Autodesk Inventor part; units mm, degrees
ref_plane "YZ Plane" through (0, 0, 0) normal (1, 0, 0) x (0, 1, 0)
ref_plane "XZ Plane" through (0, 0, 0) normal (0, 1, 0) x (-1, 0, 0)
ref_plane "XY Plane" through (0, 0, 0) normal (0, 0, 1) x (1, 0, 0)
sketch "Schizzo1" plane through (0, 0, 0) normal (0, 0, 1) x (1, 0, 0)
  line L0 (50, -12.5) -> (-50, -12.5)
  line L1 (-50, -12.5) -> (-50, 12.5)
  line L2 (-50, 12.5) -> (50, 12.5)
  line L3 (50, 12.5) -> (50, -12.5)
  line L4 (50, -12.5) -> (-50, 12.5) construction
  line L5 (-50, -12.5) -> (50, 12.5) construction
  point P0 (0, 0)
  dimension "d0" = 100
  dimension "d1" = 25
extrude "Estrusione1" add sketch "Schizzo1" along normal blind 15
sketch "Schizzo2" plane through (-50, 12.5, 0) normal (0, 1, 0) x (1, 0, 0)
  line L0 (50, 0) -> (50, 1)
  line L1 (50, 0) -> (51, 0) construction
  circle A0 centre (50, 1) radius 9.5
  dimension "d4" = 1
  dimension "d5" = 90
  dimension "d6" = 19
extrude "Estrusione2" cut sketch "Schizzo2" against normal blind 5
sketch "Schizzo3" plane through (-50, 7.5, 0) normal (0, 1, 0) x (1, 0, 0)
  line L0 (50, 0) -> (50, 1)
  line L1 (50, 0) -> (51, 0) construction
  circle A0 centre (50, 1) radius 4
  dimension "d9" = 1
  dimension "d10" = 90
  dimension "d11" = 8
extrude "Estrusione3" cut sketch "Schizzo3" against normal blind 20
sketch "Schizzo4" plane through (0, 0, 15) normal (0, 0, 1) x (1, 0, 0)
  line L0 (-25, 0) -> (25, 0)
  line L1 (-25, 0) -> (25, 0) construction
  line L2 (50, 12.5) -> (-50, 12.5)
  point P0 (0, 0)
  point P1 (0, 0)
  dimension "d14" = 50
  dimension "d15" = 0
hole "Foro1" at (-25, 0, 15) at (25, 0, 15) direction (0, 0, -1) diameter 5.9 end through all
sketch "Schizzo5" plane through (-50, 12.5, 15) normal (0, 1, 0) x (1, 0, 0)
  circle A0 centre (50, 15) radius 23
  line L0 (100, 0) -> (0, 0)
  line L1 (67.4356, 0) -> (32.5644, 0)
  point P0 (50, 15)
  dimension "d23" = 46
extrude "Estrusione4" add sketch "Schizzo5" against normal blind 25 contours L0 A0 picked at (45.5796, -1.264)
properties part number "20_Base_Sopra" material "PLA(Stampato)(D0,646)"
Part model, mm, in its own coordinate system. A direction names the side the tool comes from. Give positions to 0.01 mm unless a question says otherwise; leave off trailing zeros. Order: outer loops, then holes, each group sorted by start corner. A loop starts at its lowest first (then second) coordinate and runs counter-clockwise, first axis right, second up. Notation, with made-up numbers: M 40,-10.5 L 49,-10.5 A12 cw 49,6.5 Z; hole C 82,44.5 d9. An arc over 180 degrees is marked long. Use a Markdown table: item, result. Add a question column.
(1) Saw through at D-D, the plane y = 8.5. Give the cut face in (x, z).
(2) Saw through at B-B, the plane x = 25. Give the cut face in (y, z).
(3) Saw through at C-C, the plane z = 11. Give the cut face in (x, y), and give its area (3 significant figures).
(4) Mould opens along X. For faces 1 (the face through (50, 0, 7)), 2 (the face through (22.513, -1.586, 7.395)), 3 (the face through (-50, 0, 7)) say: +X half, -X half, draft (parallel to the pull), parting line (faces both ways), or undercut.
(5) Drop flat-ended pins along their axis: P1, Ø12.5, axis at x = -28.5, y = 1.5, coming from the +Z side; P2, Ø3, axis at y = 8, z = 19.5, coming from the +X side; P3, Ø4, axis at x = -8.5, y = 5.5, coming from the +Z side. Give the stop position or say it passes through.
(6) Probe line 1 along X through (y, z) = (0, 6); line 2 along Y through (x, z) = (-25, 8.5); line 3 along Z through (x, y) = (-19, 3.5). List the from-to ranges inside material, lowest first. Write a range as [from, to].
(7) 3-axis set-ups, long thin cutter, end or side, ignore diameter. For faces 4 (the face through (-0.19, 10.04, 8.5)), 5 (the face through (-34, 0, 15)), 6 (the face through (33, 0, 15)): which of +Z, -Z, +X, -X, +Y, -Y reach the whole face in a straight line?
(8) Saw through at A-A, the plane y = 0. Give the cut face in (x, z), and give its area (3 significant figures).
Answer key:
| question | item | result |
|---|---|---|
| 1 | outline | M -50,0 L -9.45,0 A9.5 cw 9.45,0 L 50,0 L 50,15 L 17.44,15 A23 ccw -17.44,15 L -50,15 Z |
| 2 | outline | M -12.5,0 L -2.95,0 L -2.95,15 L -12.5,15 Z; M 2.95,0 L 12.5,0 L 12.5,15 L 2.95,15 Z |
| 3 | outline | M -50,-12.5 L 50,-12.5 L 50,12.5 L -50,12.5 Z; hole C -25,0 d5.9; hole C 25,0 d5.9 |
| 3 | area | 2,450 mm^2 |
| 4 | face 1 | +X half |
| 4 | face 2 | undercut |
| 4 | face 3 | -X half |
| 5 | P1 | z = 15 |
| 5 | P2 | x = 14.32 |
| 5 | P3 | z = 22.06 |
| 6 | line 1 | [-50, -27.95], [-22.05, 22.05], [27.95, 50] |
| 6 | line 2 | [-12.5, -2.95], [2.95, 12.5] |
| 6 | line 3 | [0, 15] |
| 7 | face 4 | -Z, +Y |
| 7 | face 5 | +Z, -X, +Y, -Y |
| 7 | face 6 | +Z, +X, +Y, -Y |
| 8 | outline | M -50,0 L -27.95,0 L -27.95,15 L -50,15 Z; M -22.05,0 L -3.87,0 A4 cw 3.87,0 L 22.05,0 L 22.05,15 L 17.44,15 A23 ccw -17.44,15 L -22.05,15 Z; M 27.95,0 L 50,0 L 50,15 L 27.95,15 Z |
| 8 | area | 1,500 mm^2 |
